Part print with two shaded views. Sizes in mm from the minimum x, y, z corner. A direction names the side the tool comes from. Round coordinates to 2 decimals unless told otherwise and drop trailing zeros. Order: outer loops, then holes, each group sorted by start corner. A loop starts at its lowest first (then second) coordinate and runs counter-clockwise, first axis right, second up. Notation, with made-up numbers: (37, 50.25) -> (47, 50.25) arc R30 cw to (47, 87.25) -> close; hole circle Ø8 at (-1, 27). An arc over 180 degrees is marked (long way). Answer as a JSON object with one key per item and string values.
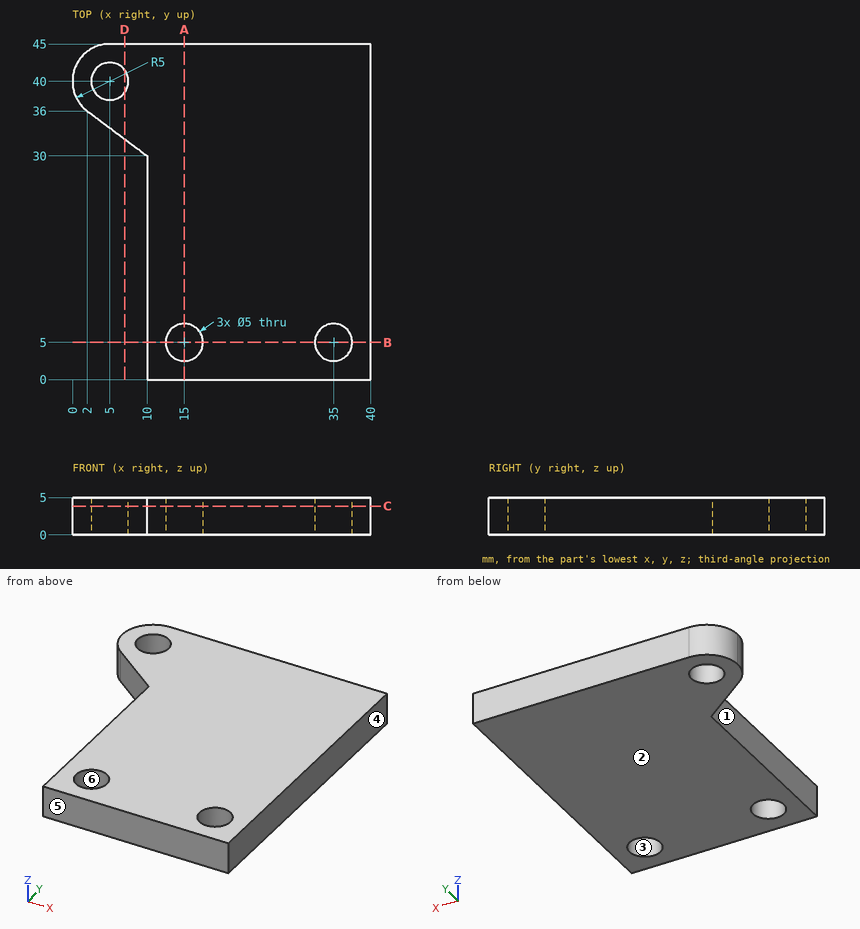
1) Which spindle directions (+Z, -Z, +X, -X, +Y, -Y) get a long thin tool onto all of the face, cutting with end or side? Do the marked faces 1 and 2. Say none if no direction does.
Checked values:
{"face 1": "+Z, -Z, -X, -Y", "face 2": "-Z, +X, -X, +Y, -Y"}
2) Probe L1, parallel to Y at x = 15, z = 3.65; L2, parallel to X at y = 29.5, z = 3.6; L3, parallel to X at y = 39, z = 2.35. List the from-to ranges inside material, lowest first. Write a range as from..to.
Checked values:
{"L1": "y = 0..2.5, 7.5..45", "L2": "x = 10..40", "L3": "x = 0.1..2.71, 7.29..40"}
3) Cut at C-C, the plane z = 3.85. Give the cut face in (x, y), plus the area to 3 significant figures.
Checked values:
{"outline": "(2, 36) -> (10, 30) -> (10, 0) -> (40, 0) -> (40, 45) -> (5, 45) arc R5 ccw to start; hole circle Ø5 at (5, 40); hole circle Ø5 at (15, 5); hole circle Ø5 at (35, 5)", "area": "1,400 mm²"}
4) Pull direction Y, two halves, no side cores. Call the marked faces 3, 4, 5 and 6: pulls with the +Y half, pulls with the -Y half, needs draft (parallel to the pull), parting line crosses it, or undercut.
Checked values:
{"face 3": "undercut", "face 4": "needs draft", "face 5": "pulls with the -Y half", "face 6": "undercut"}
5) Cut at B-B, the plane y = 5. Give the cut face in (x, z).
Checked values:
{"outline": "(10, 0) -> (12.5, 0) -> (12.5, 5) -> (10, 5) -> close; (17.5, 0) -> (32.5, 0) -> (32.5, 5) -> (17.5, 5) -> close; (37.5, 0) -> (40, 0) -> (40, 5) -> (37.5, 5) -> close"}
6) Cut at A-A, the plane x = 15. Give the cut face in (y, z), plus the area to 3 significant figures.
Checked values:
{"outline": "(0, 0) -> (2.5, 0) -> (2.5, 5) -> (0, 5) -> close; (7.5, 0) -> (45, 0) -> (45, 5) -> (7.5, 5) -> close", "area": "200 mm²"}
7) Flat gauge pins, fed straight in: pin 1 Ø1 at (x, z) = (5.5, 2.5) entering from -Y; pin 2 Ø3 at (x, y) = (5, 40) entering from +Z. Where does each tip first touch, or does it go through?
Checked values:
{"pin 1": "stops at y = 33", "pin 2": "passes through"}
8) Cut at D-D, the plane x = 7. Give the cut face in (y, z), plus the area to 4 significant figures.
Checked values:
{"outline": "(32.25, 0) -> (38.5, 0) -> (38.5, 5) -> (32.25, 5) -> close; (41.5, 0) -> (45, 0) -> (45, 5) -> (41.5, 5) -> close", "area": "48.75 mm²"}
